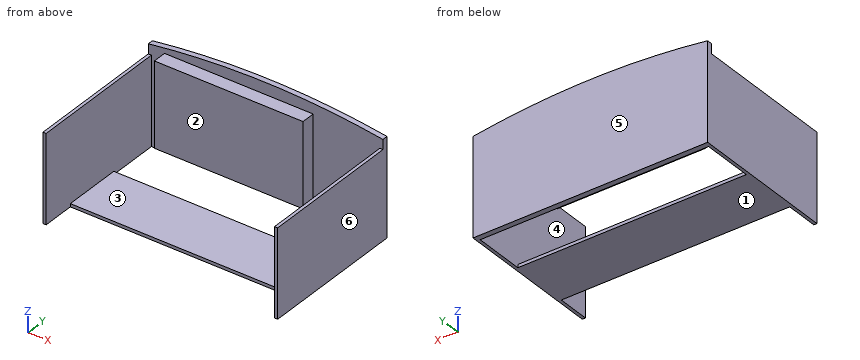
```python
from build123d import *

# Parameters (mm, degrees)
BOSS_EXTRUDE1_DEPTH = 28
SKETCH2_W           = 16
SKETCH2_H           = 450
BOSS_EXTRUDE2_DEPTH = 727
SKETCH3_W           = 16
SKETCH3_H           = 300
BOSS_EXTRUDE3_DEPTH = 1168
SKETCH4_W           = 760
SKETCH4_H           = 430
BOSS_EXTRUDE4_DEPTH = 70


with BuildPart() as part:
    # Sketch1 → Boss-Extrude1 (new body)
    with BuildSketch(Plane(origin=(0, 0, 0), x_dir=(1, 0, 0), z_dir=(0, 1, 0))):
        with BuildLine():
            Line((-600, -250), (-600, 250))
            Line((-600, 250), (600, 250))
            Line((600, 250), (600, -250))
            ThreePointArc((600, -250), (0, -295), (-600, -250))
        make_face()
    extrude(amount=BOSS_EXTRUDE1_DEPTH)

    # Sketch2 → Boss-Extrude2 (add)
    with BuildSketch(Plane.XZ):
        with Locations((-592, -25)):
            Rectangle(SKETCH2_W, SKETCH2_H)
    boss_extrude2 = extrude(amount=BOSS_EXTRUDE2_DEPTH)

    # Mirror1: Boss-Extrude2 across plane
    add(boss_extrude2.mirror(Plane(origin=(0, 0, 0), x_dir=(0, 0, 1), z_dir=(1, 0, 0))))

    # Sketch3 → Boss-Extrude3 (add)
    with BuildSketch(Plane(origin=(-584, 0, 0), x_dir=(0, 0, -1), z_dir=(1, 0, 0))):
        with Locations((242, -410)):
            Rectangle(SKETCH3_W, SKETCH3_H)
    extrude(amount=BOSS_EXTRUDE3_DEPTH)

    # Sketch4 → Boss-Extrude4 (add)
    with BuildSketch(Plane.XZ):
        with Locations((-137, 20)):
            Rectangle(SKETCH4_W, SKETCH4_H)
    extrude(amount=BOSS_EXTRUDE4_DEPTH)


solid = part.part
```
Geometry check sheet. Reference: the model listing, model coordinates, mm. Face numbers are marked on the shaded views. A direction names the side the tool comes from. Coordinates: 2 decimals unless noted, no trailing zeros. Loops run counter-clockwise (first coordinate to the right, second up) from the corner with the lowest first, then second, coordinate; pieces in that order, holes last.
Item 1: Sectioned sample at D-D, the plane x = 67. Record the boundary of the cut face in (y, z), then the cut area to 3 significant figures.
Item 2: Thickness scan on line 1 (X direction, y = -451, z = 81.5); line 2 (Z direction, x = -278, y = -3); line 3 (Z direction, x = 302, y = -285). Record the ranges inside material, lowest first.
Item 3: Sectioned sample at C-C, the plane y = -155. Record the boundary of the cut face in (x, z), then the cut area to 3 significant figures.
Item 4: Release check for a two-part mould opening along X. For the marked faces 4, 5 and 6 record: released by +X, released by -X, zero draft, split by the parting line, or undercut.
Item 5: Sectioned sample at A-A, the plane y = -52.5. Record the boundary of the cut face in (x, z).
Item 6: Sectioned sample at B-B, the plane z = -137. Record the boundary of the cut face in (x, y).
Item 7: Access from +Z, -Z, +X, -X, +Y, -Y to the whole of each face (thin tool, end or side, straight path). Record for the marked faces 1, 2 and 3.
Item 8: Go/stop test with flat-tipped pins: pin 1 Ø1.5 at (x, z) = (330.5, 113.5) entering from -Y; pin 2 Ø21 at (x, y) = (-108.5, -36.5) entering from -Z; pin 3 Ø13 at (x, y) = (-593.5, -384) entering from +Z. Record where each tip stops, or that it passes through.
Check result:
1. outline: (-560, -250) - (-260, -250) - (-260, -234) - (-560, -234) - close; (-70, -195) - (0, -195) - (0, -250) - (28, -250) - (28, 294.44) - (0, 294.44) - (0, 235) - (-70, 235) - close
1. area: 50,100 mm2
2. line 1: x = -600 to -584, 584 to 600
2. line 2: z = -195 to 235
2. line 3: z = -250 to -234
3. outline: (-600, -250) - (-584, -250) - (-584, 200) - (-600, 200) - close; (584, -250) - (600, -250) - (600, 200) - (584, 200) - close
3. area: 14,400 mm2
4. face 4: undercut
4. face 5: zero draft
4. face 6: released by +X
5. outline: (-600, -250) - (-584, -250) - (-584, 200) - (-600, 200) - close; (-517, -195) - (243, -195) - (243, 235) - (-517, 235) - close; (584, -250) - (600, -250) - (600, 200) - (584, 200) - close
6. outline: (-600, -727) - (-584, -727) - (-584, 0) - (-517, 0) - (-517, -70) - (243, -70) - (243, 0) - (584, 0) - (584, -727) - (600, -727) - (600, 28) - (-600, 28) - close
7. face 1: -Z, +X, -X, +Y, -Y
7. face 2: +Z, -Z, -Y
7. face 3: +Z, -Y
8. pin 1: stops at y = 0
8. pin 2: stops at z = -195
8. pin 3: stops at z = 200
